Build history of the part. All positions in model axes, mm. A direction names the side the tool comes from. Coordinates: 2 decimals unless noted, no trailing zeros. Order: outer loops, then holes, each group sorted by start corner. A loop starts at its lowest first (then second) coordinate and runs counter-clockwise, first axis right, second up. Notation, with made-up numbers: (-15.5, -3) - (12.5, -3) arc R15 ccw to (12.5, 7) - close; hole circle Ø9 at (64, 25). An arc over 180 degrees is marked (long way). Write each question's results on one line, items separated by ' | '.
Autodesk Inventor part; units mm, degrees
ref_plane "YZ Plane" through (0, 0, 0) normal (1, 0, 0) x (0, 1, 0)
ref_plane "XZ Plane" through (0, 0, 0) normal (0, 1, 0) x (-1, 0, 0)
ref_plane "XY Plane" through (0, 0, 0) normal (0, 0, 1) x (1, 0, 0)
sketch "スケッチ1" plane through (0, 0, 0) normal (1, 0, 0) x (0, 1, 0)
  circle A0 centre (0, 0) radius 2
  dimension "d0" = 4
extrude "押し出し1" add sketch "スケッチ1" along normal blind 64
sketch "スケッチ4" plane through (0, 0, 0) normal (-1, 0, 0) x (0, 0, 1)
  circle A0 centre (0, 0) radius 1.5
  dimension "d16" = 3
extrude "押し出し2" add sketch "スケッチ4" along normal blind 8
sketch "スケッチ5" plane through (64, 0, 0) normal (1, 0, 0) x (0, 0, -1)
  circle A0 centre (0, 0) radius 1.5
  dimension "d19" = 3
extrude "押し出し3" add sketch "スケッチ5" along normal blind 8
thread "ねじ1"
thread "ねじ2"
sketch "スケッチ2" plane through (64, 0, 0) normal (1, 0, 0) x (0, 0, -1)
  circle A0 centre (0, 0) radius 2
  line L0 (0, -2.8) -> (0, 2.8)
  point P0 (0, 2)
ref_plane "作業平面1" through (64, 2, 0) normal (0, 1, 0) x (-1, 0, 0)
sketch "スケッチ3" plane through (64, 2, 0) normal (0, 1, 0) x (-1, 0, 0)
  line L0 (64, 0) -> (0, 0)
  line L1 (0, 2) -> (0, -2)
  line L2 (-8, 1.5) -> (-8, -1.5)
  line L3 (72, -1.5) -> (72, 1.5)
  point P0 (4.5, 0)
  point P1 (59.5, 0)
  dimension "d22" = 12.5
  dimension "d23" = 12.5
hole "穴1" at (59.5, 2, 0) at (4.5, 2, 0) direction (0, -1, 0) diameter 2 end through all
properties part number "GearShaft_1" material "鉄、鋳鉄"
1. Band-saw the part on C-C on x = 4.5. Give the cut face in (y, z).
Solved:
outline: (-1.73, -1) arc R2 ccw to (1.73, -1) - close; (-1.73, 1) - (1.73, 1) arc R2 ccw to start
2. Probe line 1 (X direction, y = -0.45, z = 0); line 2 (X direction, y = 0.45, z = -0.65); line 3 (Z direction, x = 4.5, y = 0.55). List the from-to ranges inside material, lowest first.
Solved:
line 1: x = -8 to 3.5, 5.5 to 58.5, 60.5 to 72 | line 2: x = -8 to 3.74, 5.26 to 58.74, 60.26 to 72 | line 3: z = -1.92 to -1, 1 to 1.92
3. Two-plate mould, pull along X, no slides. Class faces 3 (the face through (-8, 0, 0)), 4 (the face through (67.94, -0.07, 1.5)), 5 (the face through (59.2, -0.028, 0.954)): +X half, -X half, draft (parallel to the pull), parting line (faces both ways), or undercut.
Solved:
face 3: -X half | face 4: draft | face 5: undercut
4. Band-saw the part on B-B on x = 56. Give the cut face in (y, z).
Solved:
outline: circle Ø4 at (0, 0)
5. Tool access for faces 1 (the face through (32, -2, 0)), 2 (the face through (-3.94, -0.07, -1.5)): list every direction of +Z, -Z, +X, -X, +Y, -Y with a clear straight run to the whole face (end or side of a thin tool).
Solved:
face 1: +X, -X | face 2: -X
6. Drop flat-ended pins along their axis: pin 1 Ø1.8 at (x, z) = (59.5, 0) entering from +Y; pin 2 Ø2 at (x, z) = (31, 0.5) entering from +Y. Give the stop position or say it passes through.
Solved:
pin 1: passes through | pin 2: stops at y = 2
7. Band-saw the part on A-A on y = 0. Give the cut face in (x, z), then the cut area to 3 significant figures.
Solved:
outline: (-8, -1.5) - (0, -1.5) - (0, -2) - (64, -2) - (64, -1.5) - (72, -1.5) - (72, 1.5) - (64, 1.5) - (64, 2) - (0, 2) - (0, 1.5) - (-8, 1.5) - close; hole circle Ø2 at (4.5, 0); hole circle Ø2 at (59.5, 0) | area: 298 mm2
